```python
from build123d import *

# Parameters (mm, degrees)
SKETCH1_W           = 46
SKETCH1_H           = 64
SKETCH1_R           = 3
SKETCH1_R_2         = 1.2
SKETCH1_R_3         = 6.35
SKETCH1_W_2         = 5
SKETCH1_H_2         = 15
SKETCH1_W_3         = 10
SKETCH1_H_3         = 17.5
BOSS_EXTRUDE1_DEPTH = 5
FILLET1_R           = 5


with BuildPart() as part:
    # Sketch1 → Boss-Extrude1 (new body)
    with BuildSketch(Plane.XY):
        with Locations((0, 32)):
            Rectangle(SKETCH1_W, SKETCH1_H)
        with Locations((16, 50)):
            Circle(SKETCH1_R, mode=Mode.SUBTRACT)
        with Locations((16, 18.2)):
            Circle(SKETCH1_R_2, mode=Mode.SUBTRACT)
        with Locations((16, 58.5)):
            Circle(SKETCH1_R_2, mode=Mode.SUBTRACT)
        with Locations((-16, 58.5)):
            Circle(SKETCH1_R_2, mode=Mode.SUBTRACT)
        with Locations((-16, 18.2)):
            Circle(SKETCH1_R_2, mode=Mode.SUBTRACT)
        with Locations((-16, 50)):
            Circle(SKETCH1_R, mode=Mode.SUBTRACT)
        with Locations((0, 14)):
            Circle(SKETCH1_R_3, mode=Mode.SUBTRACT)
        with Locations((16, 32.5)):
            Rectangle(SKETCH1_W_2, SKETCH1_H_2, mode=Mode.SUBTRACT)
        with Locations((2.5, 44.25)):
            Rectangle(SKETCH1_W_3, SKETCH1_H_3, mode=Mode.SUBTRACT)
        with Locations((-16, 32.5)):
            Rectangle(SKETCH1_W_2, SKETCH1_H_2, mode=Mode.SUBTRACT)
    extrude(amount=BOSS_EXTRUDE1_DEPTH)

    # Fillet1
    fillet1_edges = [part.edges().sort_by_distance(p)[0] for p in [
        (23, 0, 2.5),
        (-23, 0, 2.5),
        (-23, 64, 2.5),
        (23, 64, 2.5),
    ]]
    fillet(fillet1_edges, radius=FILLET1_R)


solid = part.part
```
The model under review builds one solid part; all positions refer to its coordinate system, in mm. A direction names the side the tool comes from. Round coordinates to 2 decimals unless told otherwise and drop trailing zeros. Write each loop counter-clockwise with the first axis right and the second up, starting at its lowest first coordinate (ties: lowest second). Pieces come first, ordered by that corner, then holes. Notation, with made-up numbers: (-39, 43) - (-19, 43) arc R14 ccw to (-19, 68) - close; hole circle Ø6 at (-38.75, -16). An arc over 180 degrees is marked (long way). Answer as CSV lines item,"result". Start each with the question number.
(1) Draft analysis for pull direction Y (two halves, no side actions). For faces 1 (the cylindrical face through (21, 1, 3)), 2 (the flat face through (0, 32, 5)), 3 (the flat face through (7.5, 44, 2)), state which applies: pulls with the +Y half, pulls with the -Y half, needs draft (parallel to the pull), parting line crosses it, or undercut.
(2) We need section C-C on x = 16. State the section outline as (y, z) points, plus the area to 3 significant figures.
(3) For faces 4 (the flat face through (23, 32, 2)), 5 (the flat face through (18.5, 32, 2)), list the 3-axis set-ups (+Z, -Z, +X, -X, +Y, -Y) from which the entire face can be reached by the end or side of a thin tool; tool diameter is ignored.
(4) To check wall thickness, follow line 1 (Y direction, x = 16, z = 3.6); line 2 (X direction, y = 37, z = 0.45); line 3 (X direction, y = 33, z = 2.6). State the ranges of each line that lie inside material, in increasing order.
(5) For pin 1 Ø3 at (x, y) = (16, 18.2) entering from +Z, flat-tipped, find the tip position at first contact; note if it passes through.
(6) We need section D-D on y = 50. State the section outline as (x, z) points, plus the area to 3 significant figures.
(7) We need section B-B on z = 0.85. Give the number of separate pieces and of enclosed holes in the cut face, plus the area to 3 significant figures.
(8) We need section A-A on y = 14. State the section outline as (x, z) points, plus the area to 4 significant figures.
Worked answers:
1,face 1,"pulls with the -Y half"
1,face 2,"needs draft"
1,face 3,"undercut"
2,outline,"(0, 0) - (17, 0) - (17, 5) - (0, 5) - close; (19.4, 0) - (25, 0) - (25, 5) - (19.4, 5) - close; (40, 0) - (47, 0) - (47, 5) - (40, 5) - close; (53, 0) - (57.3, 0) - (57.3, 5) - (53, 5) - close; (59.7, 0) - (64, 0) - (64, 5) - (59.7, 5) - close"
2,area,"191 mm²"
3,face 4,"+Z, -Z, +X, +Y, -Y"
3,face 5,"+Z, -Z"
4,line 1,"0 to 17, 19.4 to 25, 40 to 47, 53 to 57.3, 59.7 to 64"
4,line 2,"-23 to -18.5, -13.5 to -2.5, 7.5 to 13.5, 18.5 to 23"
4,line 3,"-23 to -18.5, -13.5 to 13.5, 18.5 to 23"
5,pin 1,"z = 5"
6,outline,"(-23, 0) - (-19, 0) - (-19, 5) - (-23, 5) - close; (-13, 0) - (-2.5, 0) - (-2.5, 5) - (-13, 5) - close; (7.5, 0) - (13, 0) - (13, 5) - (7.5, 5) - close; (19, 0) - (23, 0) - (23, 5) - (19, 5) - close"
6,area,"120 mm²"
7,separate pieces,"1"
7,enclosed holes,"10"
7,area,"2,400 mm²"
8,outline,"(-23, 0) - (-6.35, 0) - (-6.35, 5) - (-23, 5) - close; (6.35, 0) - (23, 0) - (23, 5) - (6.35, 5) - close"
8,area,"166.5 mm²"
